from build123d import *
from build123d.topology import SkipClean

# Parameters (mm, degrees)
SKETCH1_R           = 20.32
BOSS_EXTRUDE1_DEPTH = 15.367
SKETCH2_R           = 19.05
CUT_EXTRUDE1_DEPTH  = 33.587566479
BOSS_EXTRUDE2_DEPTH = 2.667
CUT_EXTRUDE2_DEPTH  = 96.144107805
SKETCH6_R           = 19.05
CUT_EXTRUDE3_DEPTH  = 96.144107805
SKETCH7_W           = 165.1
SKETCH7_H           = 177.8
SKETCH7_R           = 66.675
BOSS_EXTRUDE3_DEPTH = 6.985
SKETCH10_W          = 165.1
SKETCH10_H          = 177.8
SKETCH10_W_2        = 148.59
SKETCH10_H_2        = 160.02
BOSS_EXTRUDE5_DEPTH = 1.905
CUT_EXTRUDE4_DEPTH  = 122.605799303
CUT_EXTRUDE5_DEPTH  = 122.641870259
FILLET1_R           = 16.51
FILLET2_R           = 11.43
CHAMFER1_SIZE       = 1.905
SKETCH13_R          = 1.905
CUT_EXTRUDE6_DEPTH  = 122.605799303
SKETCH14_R          = 3.175
CUT_EXTRUDE7_DEPTH  = 3.175


with BuildPart() as part:
    # Sketch1 → Boss-Extrude1 (new body)
    with BuildSketch(Plane(origin=(0, 0, 0), x_dir=(1, 0, 0), z_dir=(0, 1, 0))):
        with Locations(Location((0, 0, 0), (0, 0, 270))):
            Circle(SKETCH1_R)
    extrude(amount=BOSS_EXTRUDE1_DEPTH)

    # Sketch2 → Cut-Extrude1 (cut, through all)
    with BuildSketch(Plane(origin=(0, 15.367, 0), x_dir=(1, 0, 0), z_dir=(0, 1, 0))):
        with Locations(Location((0, 0, 0), (0, 0, 270))):
            Circle(SKETCH2_R)
    extrude(amount=-CUT_EXTRUDE1_DEPTH, mode=Mode.SUBTRACT)

    # Sketch3 → Boss-Extrude2 (add)
    with BuildSketch(Plane(origin=(0, 0, 0), x_dir=(1, 0, 0), z_dir=(0, 1, 0))):
        with BuildLine():
            ThreePointArc((64.909922392, 15.24), (41.409109052, 52.25745222), (0, 66.675))
            Line((0, 66.675), (0, 34.925))
            ThreePointArc((0, 34.925), (-14.514994402, 31.765871033), (-26.404091066, 22.86))
            Line((-26.404091066, 22.86), (-57.15, 34.342875899))
            ThreePointArc((-57.15, 34.342875899), (-66.644798483, -2.006604135), (-54.980293415, -37.719))
            Line((-54.980293415, -37.719), (-29.91080298, -18.030515524))
            ThreePointArc((-29.91080298, -18.030515524), (11.688528505, -32.911000082), (34.583107671, 4.874862956))
            Line((34.583107671, 4.874862956), (64.909922392, 15.24))
        make_face()
    extrude(amount=BOSS_EXTRUDE2_DEPTH)

    # Sketch4 → Cut-Extrude2 (cut, through all)
    with SkipClean():  # the faces are left unmerged after this step: merging them gives an invalid solid
        with BuildSketch(Plane(origin=(0, 2.667, 0), x_dir=(1, 0, 0), z_dir=(0, 1, 0))):
            with BuildLine():
                Line((-29.91080298, -18.030515524), (-18.272118104, -8.89))
                ThreePointArc((-18.272118104, -8.89), (4.561412069, -19.801412069), (20.32, 0))
                Line((20.32, 0), (34.583107671, 4.874862956))
                ThreePointArc((34.583107671, 4.874862956), (15.066975095, -42.423579526), (-29.91080298, -18.030515524))
            make_face()
        extrude(amount=-CUT_EXTRUDE2_DEPTH, mode=Mode.SUBTRACT)

    # Sketch6 → Cut-Extrude3 (cut, through all)
    with SkipClean():  # the faces are left unmerged after this step: merging them gives an invalid solid
        with BuildSketch(Plane(origin=(0, 2.667, 0), x_dir=(1, 0, 0), z_dir=(0, 1, 0))):
            with Locations(Location((0, 0, 0), (0, 0, 270))):
                Circle(SKETCH6_R)
        extrude(amount=-CUT_EXTRUDE3_DEPTH, mode=Mode.SUBTRACT)

    # Sketch7 → Boss-Extrude3 (add)
    with SkipClean():  # the faces are left unmerged after this step: merging them gives an invalid solid
        with BuildSketch(Plane(origin=(0, 0, 0), x_dir=(1, 0, 0), z_dir=(0, 1, 0))):
            Rectangle(SKETCH7_W, SKETCH7_H)
            with Locations(Location((0, 0, 0), (0, 0, 90))):
                Circle(SKETCH7_R, mode=Mode.SUBTRACT)
        extrude(amount=BOSS_EXTRUDE3_DEPTH)

    # Sketch10 → Boss-Extrude5 (add)
    with SkipClean():  # the faces are left unmerged after this step: merging them gives an invalid solid
        with BuildSketch(Plane(origin=(0, 6.985, 0), x_dir=(1, 0, 0), z_dir=(0, 1, 0))):
            Rectangle(SKETCH10_W, SKETCH10_H)
            Rectangle(SKETCH10_W_2, SKETCH10_H_2, mode=Mode.SUBTRACT)
        extrude(amount=BOSS_EXTRUDE5_DEPTH)

    # Sketch11 → Cut-Extrude4 (cut, through all)
    with SkipClean():  # the faces are left unmerged after this step: merging them gives an invalid solid
        with BuildSketch(Plane(origin=(0, 6.985, 0), x_dir=(1, 0, 0), z_dir=(0, 1, 0))):
            with BuildLine():
                Line((64.909922392, 15.24), (82.55, 15.24))
                ThreePointArc((82.55, 15.24), (103.174054638, -85.896323799), (0, -88.9))
                Line((0, -88.9), (0, -66.675))
                ThreePointArc((0, -66.675), (26.234384866, -20.788279139), (64.909922392, 15.24))
            make_face()
        extrude(amount=-CUT_EXTRUDE4_DEPTH, mode=Mode.SUBTRACT)

    # Sketch12 → Cut-Extrude5 (cut, through all)
    with SkipClean():  # the faces are left unmerged after this step: merging them gives an invalid solid
        with BuildSketch(Plane(origin=(0, 8.89, 0), x_dir=(1, 0, 0), z_dir=(0, 1, 0))):
            with BuildLine():
                Line((74.295, 15.24), (82.55, 15.24))
                ThreePointArc((82.55, 15.24), (101.289385527, -84.402378772), (0, -88.9))
                Line((0, -88.9), (0, -80.01))
                ThreePointArc((0, -80.01), (30.780955415, -27.419095223), (74.295, 15.24))
            make_face()
        extrude(amount=-CUT_EXTRUDE5_DEPTH, mode=Mode.SUBTRACT)

    # Fillet1
    fillet1_edges = [part.edges().sort_by_distance(p)[0] for p in [
        (82.55, 3.4925, -88.9),
        (-82.55, 3.4925, -88.9),
        (-82.55, 3.4925, 88.9),
    ]]
    fillet(fillet1_edges, radius=FILLET1_R)

    # Fillet2
    fillet2_edges = [part.edges().sort_by_distance(p)[0] for p in [
        (74.295, 7.9375, -80.01),
        (-74.295, 7.9375, -80.01),
        (-74.295, 7.9375, 80.01),
    ]]
    fillet(fillet2_edges, radius=FILLET2_R)

    # Chamfer1
    chamfer1_edges = [part.edges().sort_by_distance(p)[0] for p in [
        (-66.675, 6.985, 0),
    ]]
    chamfer(chamfer1_edges, length=CHAMFER1_SIZE)

    # Sketch13 → Cut-Extrude6 (cut, through all)
    with SkipClean():  # the faces are left unmerged after this step: merging them gives an invalid solid
        with BuildSketch(Plane(origin=(0, 6.985, 0), x_dir=(1, 0, 0), z_dir=(0, 1, 0))):
            with Locations(Location((63.5, 71.12, 0), (0, 0, 270))):
                Circle(SKETCH13_R)
            with Locations(Location((-63.5, 71.12, 0), (0, 0, 270))):
                Circle(SKETCH13_R)
            with Locations(Location((-63.5, -71.12, 0), (0, 0, 270))):
                Circle(SKETCH13_R)
        extrude(amount=-CUT_EXTRUDE6_DEPTH, mode=Mode.SUBTRACT)

    # Sketch14 → Cut-Extrude7 (cut)
    with SkipClean():  # the faces are left unmerged after this step: merging them gives an invalid solid
        with BuildSketch(Plane(origin=(0, 6.985, 0), x_dir=(1, 0, 0), z_dir=(0, 1, 0))):
            with Locations(Location((49.53, 58.42, 0), (0, 0, 270))):
                Circle(SKETCH14_R)
        extrude(amount=-CUT_EXTRUDE7_DEPTH, mode=Mode.SUBTRACT)


solid = part.part
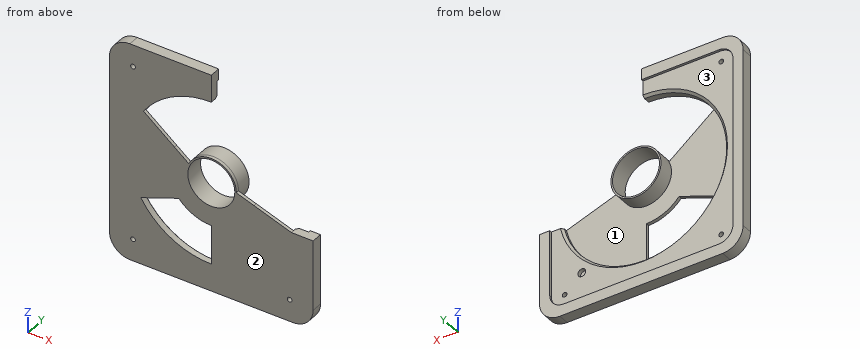
CAD build for the part. Positions are in the model's coordinates, mm. Face numbers are marked on the shaded views. Round coordinates to 2 decimals unless told otherwise and drop trailing zeros. Return JSON: item names as keys, results as strings.
(1) Pin check, flat tips, straight feed: pin 1 Ø7.5 at (x, z) = (49.53, -58.42) entering from +Y (3 decimals); pin 2 Ø12 at (x, z) = (13.5, 25) entering from +Y; pin 3 Ø3 at (y, z) = (6.5, -11) entering from +X; pin 4 Ø2.5 at (y, z) = (5.5, 82) entering from +X. Stop position of each tip, or through.
Answer key:
{"pin 1": "stops at y = 6.985", "pin 2": "passes through", "pin 3": "stops at x = 17.96", "pin 4": "stops at x = 0"}
(2) Pull direction X, two halves, no side cores. Call the marked faces 1, 2 and 3: +X half, -X half, draft (parallel to the pull), parting line (faces both ways), or undercut.
Answer key:
{"face 1": "undercut", "face 2": "draft", "face 3": "undercut"}
(3) Wall check: probe 1 along X at (y, z) = (3.3, 0) (3 decimals); probe 2 along X at (y, z) = (3.5, -71.12) (3 decimals); probe 3 along Z at (x, y) = (-14, 6). Give the ranges that are in metal, low to high. Write a range as from..to.
Answer key:
{"probe 1": "x = -82.55..-66.675, -20.32..-19.05, 19.05..20.32", "probe 2": "x = -82.55..-65.405, -61.595..61.595, 65.405..82.55", "probe 3": "z = -88.9..-66.13, -14.73..-12.92, 12.92..14.73, 66.13..88.9"}
(4) Cut at A-A (x = -45). State how many separate pieces and enclosed holes the cut face has, then the cut area to 3 significant figures.
Answer key:
{"separate pieces": "3", "enclosed holes": "0", "area": "743 mm^2"}
